Geometry: final body of the model. Coordinates: model frame, mm. Round coordinates to 2 decimals unless told otherwise and drop trailing zeros. Write each loop counter-clockwise with the first axis right and the second up, starting at its lowest first coordinate (ties: lowest second). Pieces come first, ordered by that corner, then holes. Notation, with made-up numbers: M -12.5,9 L -6.5,9 A8 cw -6.5,14 Z; hole C 81.5,9.5 d4. An arc over 180 degrees is marked long. Answer as CSV lines item,"result". Start each with the question number.
Q1. Ray query, probe 1 along Z at (x, y) = (1.25, -11.5); probe 2 along X at (y, z) = (-10.5, -2.5); probe 3 along Z at (x, y) = (0.5, -3). Return the intervals inside material, ascending.
Q2. Section query A-A on y = -11.75. Output: boundary loops of the cut face in (x, z).
Q3. First-contact query: pin 1 (2 mm diameter, centred on x = 2, z = -2.5, fed in from -Y); pin 2 (2 mm diameter, centred on x = -0.5, y = -3.5, fed in from +Z). Flat tips, straight axial feed; report the tip coordinate or a pass-through.
Q4. Section query B-B on x = -1.25. Output: boundary loops of the cut face in (y, z).
```python
from build123d import *

# Parameters (mm, degrees)
F1_DEPTH = 14
F2_SIZE  = 0.5


with BuildPart() as f1:
    # F0 (on Front) → F1 (new body)
    with BuildSketch(Plane.XZ):
        Polygon((3, -1.732051), (3, 1.732051), (0, 3.464102), (-3, 1.732051), (-3, -1.732051), (0, -3.464102), align=None)
    extrude(amount=F1_DEPTH)

    # F2
    f2_edges = [f1.edges().sort_by_distance(p)[0] for p in [
        (-1.5, -14, 2.598076),
        (-3, -14, 0),
        (-1.5, -14, -2.598076),
        (1.5, -14, -2.598076),
        (3, -14, 0),
        (1.5, -14, 2.598076),
    ]]
    chamfer(f2_edges, length=F2_SIZE)


solid = f1.part
```
Entries:
1,probe 1,"z = -2.74 to 2.74"
1,probe 2,"x = -1.67 to 1.67"
1,probe 3,"z = -3.18 to 3.18"
2,outline,"M -3,-1.73 L 0,-3.46 L 3,-1.73 L 3,1.73 L 0,3.46 L -3,1.73 Z"
3,pin 1,"stops at y = -14"
3,pin 2,"stops at z = 3.46"
4,outline,"M -14,-2.17 L -13.5,-2.74 L 0,-2.74 L 0,2.74 L -13.5,2.74 L -14,2.17 Z"
